from build123d import *

# Parameters (mm, degrees)
F3_DEPTH = 19.99
F4_R     = 8
F5_DEPTH = 1


with BuildPart() as f1:
    # F0 (on Front) → F1 (revolve)
    with BuildSketch(Plane.XZ):
        with BuildLine():
            Line((0, 90), (0, 0))
            Line((0, 0), (30, 0))
            Line((30, 0), (30, 6.5))
            ThreePointArc((30, 6.5), (26.5, 10), (30, 13.5))
            Line((30, 13.5), (30, 20))
            Line((30, 20), (15, 20))
            Line((15, 20), (15, 70))
            Line((15, 70), (30, 70))
            Line((30, 70), (30, 90))
            Line((30, 90), (0, 90))
        make_face()
    revolve(axis=Axis((0, 0, 45), (0, 0, 1)))

    # F2 (on face) → F3 (cut)
    with BuildSketch(Plane.XY.offset(90)):
        with BuildLine():
            ThreePointArc((20, 0), (19.923894, 1.743115), (19.696155, 3.472964))
            ThreePointArc((19.696155, 3.472964), (14.142136, 14.142136), (3.472964, 19.696155))
            ThreePointArc((3.472964, 19.696155), (0, 20), (-3.472964, 19.696155))
            ThreePointArc((-3.472964, 19.696155), (-14.142136, -14.142136), (19.696155, -3.472964))
            ThreePointArc((19.696155, -3.472964), (19.923894, -1.743115), (20, 0))
        make_face()
    extrude(amount=-F3_DEPTH, mode=Mode.SUBTRACT)

    # F4
    f4_edges = [f1.edges().sort_by_distance(p)[0] for p in [
        (-15, 0, 20),
        (-15, 0, 70),
        (15, 0, 45),
    ]]
    fillet(f4_edges, radius=F4_R)

    # F2 (on face) → F5 (join)
    with BuildSketch(Plane.XY.offset(90)):
        with BuildLine():
            Line((3.472964, 19.696155), (5.209445, 29.544233))
            ThreePointArc((5.209445, 29.544233), (0, 30), (-5.209445, 29.544233))
            Line((-5.209445, 29.544233), (-3.472964, 19.696155))
            ThreePointArc((-3.472964, 19.696155), (0, 20), (3.472964, 19.696155))
        make_face()
    extrude(amount=F5_DEPTH)


solid = f1.part
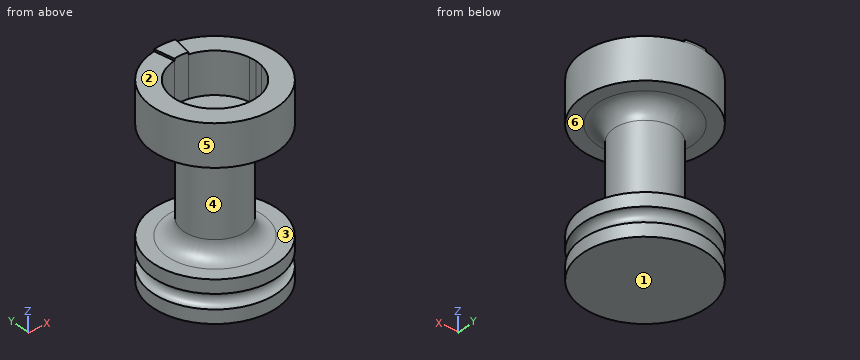
Geometry: final body of the model. Coordinates: model frame, mm. Face numbers are marked on the shaded views. A direction names the side the tool comes from. Round coordinates to 2 decimals unless told otherwise and drop trailing zeros. Loops run counter-clockwise (first coordinate to the right, second up) from the corner with the lowest first, then second, coordinate; pieces in that order, holes last. Notation, with made-up numbers: (15.5, 11.25) -> (53.5, 11.25) arc R24 ccw to (53.5, 22.25) -> close; hole circle Ø5 at (22, -24.75). An arc over 180 degrees is marked (long way). One line per question, with ' | ' between items. Start each with the question number.
1. Section B-B on y = 26.5. Count the separate pieces of the cut face and the enclosed holes in it, and give its area (3 significant figures).
2. Line query: line 1 along X through (y, z) = (0, 84); line 2 along Z through (x, y) = (-1, 25.5); line 3 along Z through (x, y) = (-23.5, -9.5). Output: solid intervals per line, ascending. Write a range as [from, to].
3. Section C-C on z = 43.5. Output: boundary loops of the cut face in (x, y), and give its area (3 significant figures).
4. Set-up query: the marked faces 5 and 6. Return all of +Z, -Z, +X, -X, +Y, -Y with unobstructed straight access to the full face (end or side cutting, diameter ignored); none if empty.
5. Mould query, pull axis Z, two halves, no side actions, for the marked faces 1, 2, 3 and 4. Classes: pulls with the +Z half, pulls with the -Z half, needs draft (parallel to the pull), parting line crosses it, or undercut.
6. Section A-A on x = 0. Output: boundary loops of the cut face in (y, z), and give its area (3 significant figures).
7. Contact query for flat-ended pins moving along their axis: pin 1 (2 mm diameter, centred on y = -2, z = 43.5, fed in from -X); pin 2 (3 mm diameter, centred on x = 23, z = 16.5, fed in from -Y); pin 3 (10 mm diameter, centred on y = 18, z = 44, fed in from -X). Output: stop coordinate, or through.
8. Section D-D on z = 10.5. Output: boundary loops of the cut face in (x, y).
Returned:
1) separate pieces: 3 | enclosed holes: 0 | area: 1,010 mm2
2) line 1: x = [-30, -20], [20, 30] | line 2: z = [0, 20], [70, 91] | line 3: z = [0, 20], [70, 90]
3) outline: circle Ø30 at (0, 0) | area: 707 mm2
4) face 5: +Z, -Z | face 6: none
5) face 1: pulls with the -Z half | face 2: pulls with the +Z half | face 3: undercut | face 4: undercut
6) outline: (-30, 0) -> (30, 0) -> (30, 6.5) arc R3.5 cw to (30, 13.5) -> (30, 20) -> (23, 20) arc R8 cw to (15, 28) -> (15, 62) arc R8 cw to (23, 70) -> (30, 70) -> (30, 91) -> (20, 91) -> (20, 70.01) -> (-20, 70.01) -> (-20, 90) -> (-30, 90) -> (-30, 70) -> (-23, 70) arc R8 cw to (-15, 62) -> (-15, 28) arc R8 cw to (-23, 20) -> (-30, 20) -> (-30, 13.5) arc R3.5 cw to (-30, 6.5) -> close | area: 3,130 mm2
7) pin 1: stops at x = -14.97 | pin 2: stops at y = -20.92 | pin 3: stops at x = -7.48
8) outline: circle Ø53.07 at (0, 0)
